```python
from build123d import *

# Parameters (mm, degrees)
PAD_DEPTH       = 9.5
CHAMFER_SIZE    = 0.5
CHAMFER001_SIZE = 0.5
CHAMFER002_SIZE = 2
CHAMFER003_SIZE = 0.5
CHAMFER004_SIZE = 2
SKETCH001_R     = 1.75
POCKET_DEPTH    = 5


with BuildPart() as part:
    # Sketch → Pad (new body)
    with BuildSketch(Plane.XY):
        Polygon((-13, 0), (0, 0), (0, 10), (4, 10), (4, 14.5), (-3, 14.5), (-3, 3), (-13, 3), align=None)
    extrude(amount=PAD_DEPTH)

    # Chamfer
    chamfer_edges = [part.edges().sort_by_distance(p)[0] for p in [
        (4, 10, 4.75),
        (4, 14.5, 4.75),
        (4, 12.25, 9.5),
        (4, 12.25, 0),
    ]]
    chamfer(chamfer_edges, length=CHAMFER_SIZE)

    # Chamfer001
    chamfer001_edges = [part.edges().sort_by_distance(p)[0] for p in [
        (1.75, 10, 0),
        (1.75, 10, 9.5),
        (0.25, 14.5, 9.5),
        (0.25, 14.5, 0),
    ]]
    chamfer(chamfer001_edges, length=CHAMFER001_SIZE)

    # Chamfer002
    chamfer002_edges = [part.edges().sort_by_distance(p)[0] for p in [
        (-3, 3, 4.75),
    ]]
    chamfer(chamfer002_edges, length=CHAMFER002_SIZE)

    # Chamfer003
    chamfer003_edges = [part.edges().sort_by_distance(p)[0] for p in [
        (0, 0, 4.75),
    ]]
    chamfer(chamfer003_edges, length=CHAMFER003_SIZE)

    # Chamfer004
    chamfer004_edges = [part.edges().sort_by_distance(p)[0] for p in [
        (-13, 1.5, 0),
        (-13, 1.5, 9.5),
    ]]
    chamfer(chamfer004_edges, length=CHAMFER004_SIZE)

    # Sketch001 (on Face5 of Chamfer004) → Pocket (cut)
    with BuildSketch(Plane(origin=(0, 3, 0), x_dir=(-1, 0, 0), z_dir=(0, 1, 0))):
        with Locations((9, 4.35)):
            Circle(SKETCH001_R)
    extrude(amount=-POCKET_DEPTH, mode=Mode.SUBTRACT)


solid = part.part
```
The listing builds one solid part. Answer for the finished solid, in the listing's coordinates (mm). A direction names the side the tool comes from. Give positions to 0.01 mm unless a question says otherwise; leave off trailing zeros. Order: outer loops, then holes, each group sorted by start corner. A loop starts at its lowest first (then second) coordinate and runs counter-clockwise, first axis right, second up.
Item 1: The part is cut by section C-C, the plane x = 0.5. Give the vertices of the cut face in (y, z), and give its area (4 significant figures).
From the geometry:
outline: (10, 0.5) - (10.5, 0) - (14, 0) - (14.5, 0.5) - (14.5, 9) - (14, 9.5) - (10.5, 9.5) - (10, 9) - close
area: 42.25 mm2
Item 2: Which of the six approach directions +Z, -Z, +X, -X, +Y, -Y give full straight-line access (tool end or side, diameter ignored) to faces 4 (the face through (-13, 2, 5)), 5 (the face through (2, 10, 5)), 6 (the face through (-3, 10, 5))?
From the geometry:
face 4: +Z, -Z, -X, +Y, -Y
face 5: +Z, -Z, +X, -Y
face 6: +Z, -Z, -X, +Y
Item 3: The part is cut by section D-D, the plane z = 1. Give the vertices of the cut face in (x, y).
From the geometry:
outline: (-12, 0) - (-0.5, 0) - (0, 0.5) - (0, 10) - (3.5, 10) - (4, 10.5) - (4, 14) - (3.5, 14.5) - (-3, 14.5) - (-3, 5) - (-5, 3) - (-12, 3) - close
Item 4: Given pin 1 Ø2 at (y, z) = (2.5, 2.5) entering from +X; pin 2 Ø4 at (x, z) = (-9, 4.35) entering from +Y, each flat-ended and moving along its own axis, determine where each tip first touches the part or whether it passes through.
From the geometry:
pin 1: stops at x = 0
pin 2: stops at y = 3
Item 5: The part is cut by section B-B, the plane x = -9. Give the vertices of the cut face in (y, z).
From the geometry:
outline: (0, 0) - (3, 0) - (3, 2.6) - (0, 2.6) - close; (0, 6.1) - (3, 6.1) - (3, 9.5) - (0, 9.5) - close
Item 6: Find the intervals of material crossed by probe 1 along Z at (x, y) = (-9, 1.5); probe 2 along X at (y, z) = (2.25, 5); probe 3 along Y at (x, z) = (3.25, 7), in increasing order.
From the geometry:
probe 1: z = 0 to 2.6, 6.1 to 9.5
probe 2: x = -13 to -10.62, -7.38 to 0
probe 3: y = 10 to 14.5
Item 7: The part is cut by section A-A, the plane z = 4.35. Give the vertices of the cut face in (x, y), and give its area (3 significant figures).
From the geometry:
outline: (-13, 0) - (-10.75, 0) - (-10.75, 3) - (-13, 3) - close; (-7.25, 0) - (-0.5, 0) - (0, 0.5) - (0, 10) - (3.5, 10) - (4, 10.5) - (4, 14) - (3.5, 14.5) - (-3, 14.5) - (-3, 5) - (-5, 3) - (-7.25, 3) - close
area: 82.6 mm2
Item 8: For a pull along X with two mould halves and no side action, classify faces 1 (the face through (0, 14.5, 5)), 2 (the face through (4, 12, 5)), 3 (the face through (-9.941, 1.521, 5.826)) as pulls with the +X half, pulls with the -X half, needs draft (parallel to the pull), parting line crosses it, or undercut.
From the geometry:
face 1: needs draft
face 2: pulls with the +X half
face 3: undercut
